Part model, mm, in its own coordinate system. Coordinates: 2 decimals unless noted, no trailing zeros. Write each loop counter-clockwise with the first axis right and the second up, starting at its lowest first coordinate (ties: lowest second). Pieces come first, ordered by that corner, then holes. Notation, with made-up numbers: (3.25, 28.5) -> (26.25, 28.5) arc R7 cw to (26.25, 40.5) -> close; hole circle Ø5 at (43.25, -7). An arc over 180 degrees is marked (long way). Write item = value, one per line.
Autodesk Inventor part; units mm, degrees
ref_plane "YZ Plane" through (0, 0, 0) normal (1, 0, 0) x (0, 1, 0)
ref_plane "XZ Plane" through (0, 0, 0) normal (0, 1, 0) x (-1, 0, 0)
ref_plane "XY Plane" through (0, 0, 0) normal (0, 0, 1) x (1, 0, 0)
sketch "Sketch1" plane through (0, 0, 0) normal (0, 0, 1) x (1, 0, 0)
  line L0 (-99, -56) -> (99, -56)
  line L1 (99, -56) -> (99, 56)
  line L2 (99, 56) -> (-99, 56)
  line L3 (-99, 56) -> (-99, -56)
  line L4 (-99, -56) -> (99, 56) construction
  line L5 (99, -56) -> (-99, 56) construction
  line L6 (-99, -56) -> (8.25, -56)
  line L7 (8.25, -56) -> (8.25, 20)
  line L8 (8.25, 20) -> (-99, 20)
  line L9 (-99, 20) -> (-99, -56)
  line L10 (8.25, 20) -> (8.25, 56)
  point P0 (0, 0)
  dimension "d0" = 112
  dimension "d1" = 198
  dimension "d3" = 76
  dimension "d50" = 8.25
extrude "Extrusion1" add sketch "Sketch1" along normal blind 1.6 contours L3 L8 L7 L0 | L7 L10 L2 L1 L0
sketch "Sketch2" plane through (0, 0, 1.6) normal (0, 0, 1) x (1, 0, 0)
  line L0 (-99, -56) -> (99, -56)
  line L1 (-99, 20) -> (-99, -56)
  line L2 (99, 56) -> (8.25, 56)
  line L3 (99, -56) -> (99, 56)
  line L4 (8.25, 20) -> (-99, 20)
  line L5 (-16.5, -52) -> (16.5, -52) construction
  line L6 (-49.5, -52) -> (-16.5, -52) construction
  point P0 (0, 0)
  point P1 (-82.5, -52)
  point P2 (49.5, -52)
  point P3 (-82.5, 52)
  point P4 (-49.5, 52)
  point P5 (-16.5, 52)
  point P6 (16.5, 52)
  point P7 (49.5, 52)
  point P8 (82.5, -52)
  point P9 (82.5, 52)
  point P10 (-33, 16)
  point P11 (0, 16)
  point P12 (0, -52)
  point P13 (-33, -52)
  point P14 (-99, 56)
  dimension "d6" = 4
  dimension "d9" = 33
  dimension "d12" = 104
  dimension "d15" = 4
  dimension "d17" = 16.5
  dimension "d18" = 16.5
  dimension "d26" = 4
hole "Hole1" at (-82.5, -52, 1.6) at (-49.5, -52, 1.6) at (-16.5, -52, 1.6) at (16.5, -52, 1.6) at (49.5, -52, 1.6) at (-82.5, 52, 1.6) at (-49.5, 52, 1.6) at (-16.5, 52, 1.6) at (16.5, 52, 1.6) at (49.5, 52, 1.6) at (82.5, -52, 1.6) at (82.5, 52, 1.6) at (-33, 16, 1.6) at (0, 16, 1.6) direction (0, 0, -1) diameter 3.4 end through all
sketch "Sketch3" plane through (0, 0, 1.6) normal (0, 0, 1) x (1, 0, 0)
  circle A0 centre (0, 16) radius 1.7
  circle A1 centre (-33, 16) radius 1.7
  circle A2 centre (82.5, 52) radius 1.7
  circle A3 centre (82.5, -52) radius 1.7
  circle A4 centre (49.5, 52) radius 1.7
  circle A5 centre (16.5, 52) radius 1.7
  circle A6 centre (49.5, -52) radius 1.7
  circle A7 centre (16.5, -52) radius 1.7
  circle A8 centre (-16.5, -52) radius 1.7
  circle A9 centre (-49.5, -52) radius 1.7
  circle A10 centre (-82.5, -52) radius 1.7
  line L0 (99, 56) -> (8.25, 56)
  line L1 (-99, 20) -> (-99, -56)
  line L2 (-99, -56) -> (99, -56)
  line L3 (99, -56) -> (99, 56)
  line L4 (99, 23) -> (0, 23) construction
  line L5 (99, 10) -> (-99, 10) construction
  line L6 (90.5, -56) -> (90.5, 10)
  line L7 (99, 23) -> (80.5, 23)
  line L8 (80.5, 23) -> (80.5, 10)
  line L9 (90.5, 10) -> (80.5, 10)
  line L10 (63.5, 10) -> (80.5, 10)
  line L11 (80.5, 10) -> (80.5, 23)
  line L12 (80.5, 23) -> (63.5, 23)
  line L13 (63.5, 23) -> (63.5, 10)
  line L14 (63.5, 10) -> (80.5, 23) construction
  line L15 (80.5, 10) -> (63.5, 23) construction
  line L16 (8.25, 56) -> (8.25, 20)
  line L17 (8.25, 20) -> (-99, 20)
  point P0 (0, 0)
  point P1 (82.5, 27)
  point P2 (72, 16.5)
  dimension "d29" = 4
  dimension "d30" = 8
  dimension "d31" = 4
  dimension "d32" = 4
  dimension "d33" = 2
  dimension "d36" = 72.5
  dimension "d37" = 17
  dimension "d38" = 13
extrude "Extrusion2" cut sketch "Sketch3" against normal through all contours L3 L2 L6 L9 L8 L7 | L8 L10 L13 L12
fillet "Fillet1" radius 8 2 edges at (-99, -56, 0.8) (99, 56, 0.8)
fillet "Fillet2" radius 2 6 edges at (90.5, 10, 0.8) (8.25, 20, 0.8) (-99, 20, 0.8) (8.25, 56, 0.8) (90.5, -56, 0.8) (99, 23, 0.8)
fillet "Fillet3" radius 1 2 edges at (63.5, 23, 0.8) (63.5, 10, 0.8)
sketch "Sketch5" plane through (0, 0, 1.6) normal (0, 0, 1) x (1, 0, 0)
  circle A0 centre (0, 16) radius 1.7
  circle A1 centre (-33, 16) radius 1.7
  circle A2 centre (82.5, 52) radius 1.7
  circle A3 centre (82.5, -52) radius 1.7
  circle A4 centre (49.5, 52) radius 1.7
  circle A5 centre (16.5, 52) radius 1.7
  circle A6 centre (49.5, -52) radius 1.7
  circle A7 centre (16.5, -52) radius 1.7
  circle A8 centre (-16.5, -52) radius 1.7
  circle A9 centre (-49.5, -52) radius 1.7
  circle A10 centre (-82.5, -52) radius 1.7
  arc A11 (88.5, -56) -> (90.5, -54) centre (88.5, -54) ccw
  line L0 (90.5, -54) -> (90.5, 8)
  arc A12 (90.5, 8) -> (88.5, 10) centre (88.5, 8) ccw
  line L1 (88.5, 10) -> (64.5, 10)
  arc A13 (63.5, 11) -> (64.5, 10) centre (64.5, 11) ccw
  line L2 (63.5, 11) -> (63.5, 22)
  arc A14 (64.5, 23) -> (63.5, 22) centre (64.5, 22) ccw
  line L3 (64.5, 23) -> (97, 23)
  line L4 (99, 25) -> (99, 48)
  arc A15 (99, 48) -> (91, 56) centre (91, 48) ccw
  line L5 (91, 56) -> (10.25, 56)
  arc A16 (10.25, 56) -> (8.25, 54) centre (10.25, 54) ccw
  line L6 (8.25, 54) -> (8.25, 22)
  arc A17 (6.25, 20) -> (8.25, 22) centre (6.25, 22) ccw
  line L7 (6.25, 20) -> (-97, 20)
  arc A18 (-97, 20) -> (-99, 18) centre (-97, 18) ccw
  line L8 (-99, 18) -> (-99, -48)
  arc A19 (-99, -48) -> (-91, -56) centre (-91, -48) ccw
  line L9 (-91, -56) -> (88.5, -56)
  arc A20 (97, 23) -> (99, 25) centre (97, 25) ccw
  point P0 (0, 0)
properties part number "Class-D RevA Board Outline"
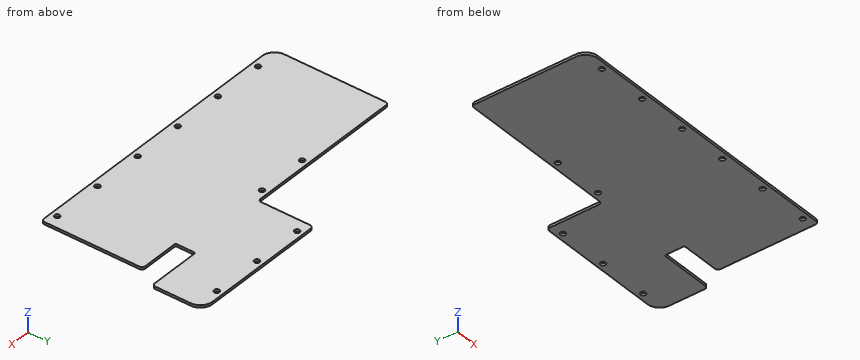
Q1. Pin check, flat tips, straight feed: pin 1 (5 mm diameter, centred on x = 13.5, y = -43, fed in from -Z); pin 2 (0.8 mm diameter, centred on y = 17, z = 1, fed in from +X); pin 3 (0.5 mm diameter, centred on y = -32.5, z = 0.5, fed in from +X); pin 4 (2.5 mm diameter, centred on x = 16.5, y = 52, fed in from +Z). Stop position of each tip, or through.
Model answer:
pin_1 = 0
pin_2 = 63.5
pin_3 = 90.5
pin_4 = through
Q2. Probe line 1 (Y direction, x = 82.5, z = 0.6); line 2 (Y direction, x = -33, z = 1.2); line 3 (Y direction, x = 49.5, z = 0.7). List the from-to ranges inside material, lowest first. Write a range as from..to.
Model answer:
line_1 = -56..-53.7, -50.3..10, 23..50.3, 53.7..56
line_2 = -56..14.3, 17.7..20
line_3 = -56..-53.7, -50.3..50.3, 53.7..56
Q3. Saw through at C-C on x = -7. Give the cut face in (y, z).
Model answer:
outline = (-56, 0) -> (20, 0) -> (20, 1.6) -> (-56, 1.6) -> close
Q4. Saw through at B-B on y = -32. Give the cut face in (x, z), and give its area (3 significant figures).
Model answer:
outline = (-99, 0) -> (90.5, 0) -> (90.5, 1.6) -> (-99, 1.6) -> close
area = 303 mm²
Q5. Saw through at A-A on z = 0.65. Count the separate pieces of the cut face and the enclosed holes in it, and give its area (3 significant figures).
Model answer:
separate_pieces = 1
enclosed_holes = 11
area = 17,200 mm²
